```python
from build123d import *

# Parameters (mm, degrees)
SKETCH_W        = 52
SKETCH_H        = 68
PAD_DEPTH       = 2
SKETCH001_W     = 48.2
SKETCH001_H     = 64.2
PAD001_DEPTH    = 1.3
SKETCH002_W     = 4.8
SKETCH002_H     = 4.8
PAD002_DEPTH    = 0.8
PAD003_DEPTH    = 64.3
SKETCH004_W     = 6
SKETCH004_H     = 52
POCKET_DEPTH    = 5
SKETCH005_W     = 7
SKETCH005_H     = 4
POCKET001_DEPTH = 1.5
POCKET002_DEPTH = 22.5
POCKET003_DEPTH = 22.5
FILLET_R        = 1.5
CHAMFER_SIZE    = 0.3
FILLET001_R     = 1


with BuildPart() as part:
    # Sketch → Pad (new body)
    with BuildSketch(Plane.XY):
        with Locations((24.25, 32.25)):
            Rectangle(SKETCH_W, SKETCH_H)
    extrude(amount=PAD_DEPTH)

    # Sketch001 (on Face6 of Pad) → Pad001 (join)
    with BuildSketch(Plane.XY.offset(2)):
        with Locations((24.25, 32.25)):
            Rectangle(SKETCH001_W, SKETCH001_H)
    extrude(amount=PAD001_DEPTH)

    # Sketch002 (on Face11 of Pad001) → Pad002 (join)
    with BuildSketch(Plane.XY.offset(3.3)):
        with Locations((1.5, 24.75)):
            Rectangle(SKETCH002_W, SKETCH002_H)
        with Locations((1.5, 39.75)):
            Rectangle(SKETCH002_W, SKETCH002_H)
    extrude(amount=PAD002_DEPTH)

    # Sketch003 (on Face9 of Pad002) → Pad003 (join)
    with BuildSketch(Plane(origin=(0, 64.35, 0), x_dir=(-1, 0, 0), z_dir=(0, 1, 0))):
        Polygon((-50.25, 0), (-52.75, 0), (-50.95359, 3.55), (-50.05359, 3.55), (-50.4, 2.95), (-50.4, 2), (-50.25, 2), align=None)
    extrude(amount=-PAD003_DEPTH)

    # Sketch004 (on Face4 of Pad003) → Pocket (cut)
    with BuildSketch(Plane(origin=(0, 0, 0), x_dir=(1, 0, 0), z_dir=(0, 0, -1))):
        with Locations((44.5, -32)):
            Rectangle(SKETCH004_W, SKETCH004_H)
    extrude(amount=-POCKET_DEPTH, mode=Mode.SUBTRACT)

    # Sketch005 (on Face24 of Pocket) → Pocket001 (cut)
    with BuildSketch(Plane.XY.offset(3.3)):
        with Locations((38.25, 59.75)):
            Rectangle(SKETCH005_W, SKETCH005_H)
    extrude(amount=-POCKET001_DEPTH, mode=Mode.SUBTRACT)

    # Sketch006 (on Face6 of Pad003) → Pocket002 (cut)
    with BuildSketch(Plane(origin=(0, 64.35, 0), x_dir=(-1, 0, 0), z_dir=(0, 1, 0))):
        Polygon((-50.25, 0), (-50.25, 3), (-49.75, 3), (-49.75, 4.5), (-53.25, 4.5), (-53.25, 0), align=None)
    extrude(amount=-POCKET002_DEPTH, mode=Mode.SUBTRACT)

    # Sketch007 (on Face21 of Pocket002) → Pocket003 (cut)
    with BuildSketch(Plane.XZ.offset(-0.05)):
        Polygon((50.25, 0), (50.25, 3), (49.75, 3), (49.75, 4.5), (53.25, 4.5), (53.25, 0), align=None)
    extrude(amount=-POCKET003_DEPTH, mode=Mode.SUBTRACT)

    # Fillet
    fillet_edges = [part.edges().sort_by_distance(p)[0] for p in [
        (50.25, -1.75, 1),
        (24.25, -1.75, 0),
        (-1.75, -1.75, 1),
        (-1.75, 32.25, 0),
        (-1.75, 66.25, 1),
        (24.25, 66.25, 0),
        (50.25, 66.25, 1),
    ]]
    fillet(fillet_edges, radius=FILLET_R)

    # Chamfer
    chamfer_edges = [part.edges().sort_by_distance(p)[0] for p in [
        (48.35, 32.25, 3.3),
    ]]
    chamfer(chamfer_edges, length=CHAMFER_SIZE)

    # Fillet001
    fillet001_edges = [part.edges().sort_by_distance(p)[0] for p in [
        (51.851795, 41.85, 1.775),
        (51.851795, 22.55, 1.775),
    ]]
    fillet(fillet001_edges, radius=FILLET001_R)


solid = part.part
```
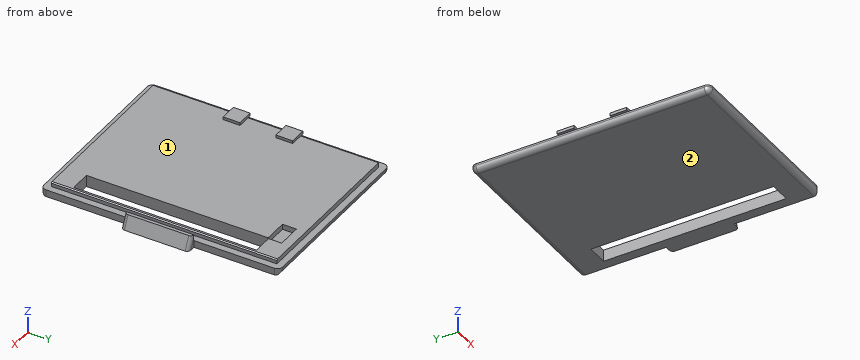
Model file for the job. Use its own axes, mm. Face numbers are marked on the shaded views. Give positions to 0.01 mm unless a question says otherwise; leave off trailing zeros. Write each loop counter-clockwise with the first axis right and the second up, starting at its lowest first coordinate (ties: lowest second). Pieces come first, ordered by that corner, then holes. Notation, with made-up numbers: M 6.5,38 L 48.5,38 A20 ccw 48.5,49 Z; hole C 16,-7 d10. An arc over 180 degrees is marked long. Use a Markdown table: item, result.
1) Cut at A-A (y = 29.5). List the corners of the cut face in (x, z), and give its area (3 significant figures).
Responses:
| item | result |
|---|---|
| outline | M -1.75,1.5 A1.5 ccw -0.25,0 L 41.5,0 L 41.5,3.3 L 0.15,3.3 L 0.15,2 L -1.75,2 Z; M 47.5,0 L 52.75,0 L 50.95,3.55 L 50.05,3.55 L 50.4,2.95 L 50.4,2 L 48.35,2 L 48.35,3 L 48.05,3.3 L 47.5,3.3 Z |
| area | 152 mm2 |
2) Pull direction X, two halves, no side cores. Call the marked faces 1 and 2: +X half, -X half, draft (parallel to the pull), parting line (faces both ways), or undercut.
Responses:
| item | result |
|---|---|
| face 1 | undercut |
| face 2 | draft |
3) Cut at C-C (y = 60.5). List the corners of the cut face in (x, z), and give its area (3 significant figures).
Responses:
| item | result |
|---|---|
| outline | M -1.75,1.5 A1.5 ccw -0.25,0 L 50.25,0 L 50.25,2 L 48.35,2 L 48.35,3 L 48.05,3.3 L 41.75,3.3 L 41.75,1.8 L 34.75,1.8 L 34.75,3.3 L 0.15,3.3 L 0.15,2 L -1.75,2 Z |
| area | 156 mm2 |
4) Pin check, flat tips, straight feed: pin 1 (1.2 mm diameter, centred on x = 36.5, y = 59.5, fed in from +Z); pin 2 (1.5 mm diameter, centred on y = 29, z = 3.5, fed in from +X); pin 3 (0.8 mm diameter, centred on y = 60.5, z = 3, fed in from -X). Stop position of each tip, or through.
Responses:
| item | result |
|---|---|
| pin 1 | stops at z = 1.8 |
| pin 2 | stops at x = 51.36 |
| pin 3 | stops at x = 0.15 |
5) Cut at B-B (x = 33). List the corners of the cut face in (y, z), and give its area (3 significant figures).
Responses:
| item | result |
|---|---|
| outline | M -1.75,1.5 A1.5 ccw -0.25,0 L 64.75,0 A1.5 ccw 66.25,1.5 L 66.25,2 L 64.35,2 L 64.35,3.3 L 0.15,3.3 L 0.15,2 L -1.75,2 Z |
| area | 218 mm2 |
6) Drill centre lines: line 1 (Y direction, x = 43, z = 1.4); line 2 (X direction, y = 35, z = 2.3); line 3 (Z direction, x = 2.5, y = 62.5). Where is each one in solid material? Low to high. Write a range as from..to.
Responses:
| item | result |
|---|---|
| line 1 | y = -1.75..6, 58..66.25 |
| line 2 | x = 0.15..41.5, 47.5..48.35, 50.4..51.59 |
| line 3 | z = 0..3.3 |
7) Cut at D-D (y = 9). List the corners of the cut face in (x, z).
Responses:
| item | result |
|---|---|
| outline | M -1.75,1.5 A1.5 ccw -0.25,0 L 41.5,0 L 41.5,3.3 L 0.15,3.3 L 0.15,2 L -1.75,2 Z; M 47.5,0 L 50.25,0 L 50.25,2 L 48.35,2 L 48.35,3 L 48.05,3.3 L 47.5,3.3 Z |
